Can you work these out from the drawing? Everything is in mm from the part's minimum corner. A direction names the side the tool comes from. Give positions to 0.01 mm unless a question says otherwise; leave off trailing zeros. Write each loop counter-clockwise with the first axis right and the second up, starting at its lowest first coordinate (ties: lowest second). Pieces come first, ordered by that corner, then holes. Notation, with made-up numbers: (13, 61.25) - (61, 61.25) arc R16 cw to (61, 82.25) - close; hole circle Ø1 at (-7, -17). An arc over 180 degrees is marked (long way). Use a Markdown table: item, result.
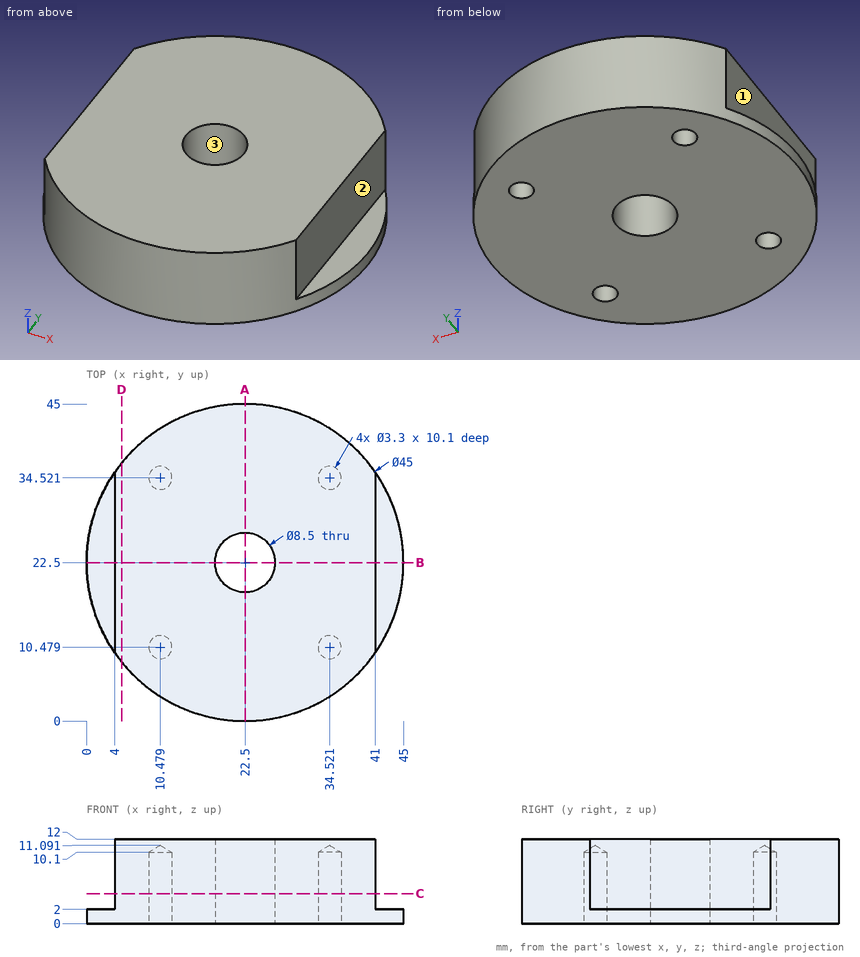
Item 1: If we section it at A-A, the plane x = 22.5: Write out the boundary of the cut face in (y, z).
Values:
| item | result |
|---|---|
| outline | (0, 0) - (18.25, 0) - (18.25, 12) - (0, 12) - close; (26.75, 0) - (45, 0) - (45, 12) - (26.75, 12) - close |
Item 2: I need wall thicknesses on line 1 along Y through (x, z) = (10.5, 9.75); line 2 along X through (y, z) = (20, 6.75) (1 decimal); line 3 along X through (y, z) = (34, 1) (1 decimal). Which ranges of each line are inside material? Lowest first, please. Write a range as [from, to].
Values:
| item | result |
|---|---|
| line 1 | y = [3.47, 8.83], [12.13, 32.87], [36.17, 41.53] |
| line 2 | x = [4, 19.1], [25.9, 41] |
| line 3 | x = [3.2, 8.9], [12, 33], [36.1, 41.8] |
Item 3: For the marked faces 1, 2 and 3, which set-ups out of +Z, -Z, +X, -X, +Y, -Y let a thin tool reach every point of the face, with its end or its side?
Values:
| item | result |
|---|---|
| face 1 | +Z, -X, +Y, -Y |
| face 2 | +Z, +X, +Y, -Y |
| face 3 | +Z, -Z |
Item 4: If we section it at B-B, the plane y = 22.5: Write out the boundary of the cut face in (x, z), plus the area to 3 significant figures.
Values:
| item | result |
|---|---|
| outline | (0, 0) - (18.25, 0) - (18.25, 12) - (4, 12) - (4, 2) - (0, 2) - close; (26.75, 0) - (45, 0) - (45, 2) - (41, 2) - (41, 12) - (26.75, 12) - close |
| area | 358 mm2 |
Item 5: Will these pins go through, and if not, where does the flat tip stop? pin 1 Ø3 at (y, z) = (23, 8.5) entering from -X; pin 2 Ø5 at (y, z) = (19, 5) entering from +X; pin 3 Ø2 at (x, z) = (13, 9) entering from -Y.
Values:
| item | result |
|---|---|
| pin 1 | stops at x = 4 |
| pin 2 | stops at x = 41 |
| pin 3 | stops at y = 1.67 |
Item 6: If we section it at D-D, the plane x = 5: Write out the boundary of the cut face in (y, z), plus the area to 3 significant figures.
Values:
| item | result |
|---|---|
| outline | (8.36, 0) - (36.64, 0) - (36.64, 12) - (8.36, 12) - close |
| area | 339 mm2 |
Item 7: If we section it at C-C, the plane z = 4.25: Write out the boundary of the cut face in (x, y), plus the area to 3 significant figures.
Values:
| item | result |
|---|---|
| outline | (4, 9.69) arc R22.5 ccw to (41, 9.69) - (41, 35.31) arc R22.5 ccw to (4, 35.31) - close; hole circle Ø3.3 at (10.48, 10.48); hole circle Ø3.3 at (10.48, 34.52); hole circle Ø8.5 at (22.5, 22.5); hole circle Ø3.3 at (34.52, 10.48); hole circle Ø3.3 at (34.52, 34.52) |
| area | 1,360 mm2 |
